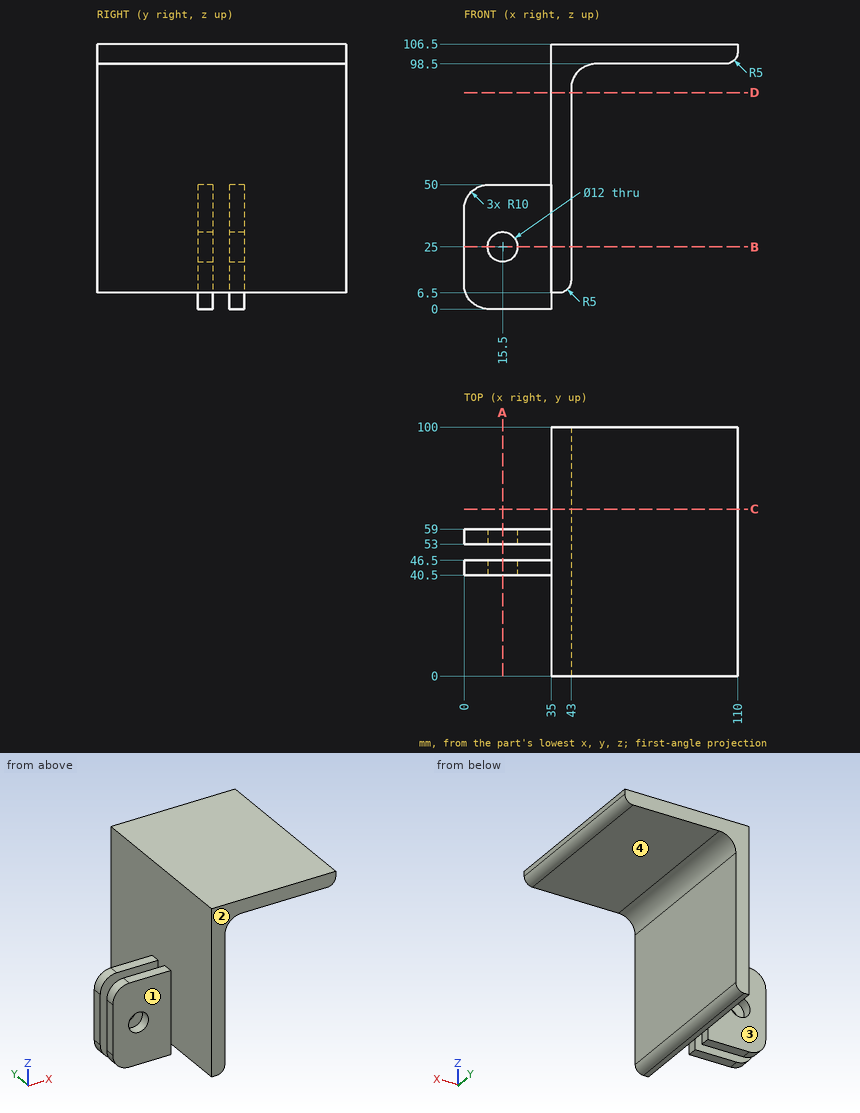
Answer from the drawing. Dimensions are ordinates in mm from the lowest x, y and z of the part. A direction names the side the tool comes from. Give positions to 0.01 mm unless a question says otherwise; leave off trailing zeros. Order: outer loops, then holes, each group sorted by start corner. A loop starts at its lowest first (then second) coordinate and runs counter-clockwise, first axis right, second up. Notation, with made-up numbers: (3.25, -6.75) -> (29.25, -6.75) arc R28 cw to (29.25, 24.25) -> close; hole circle Ø1 at (64.25, 4). An arc over 180 degrees is marked (long way). One line per item, written item: value. Start each with the question number.
(1) Flat-ended cylindrical pins translate along their axes: P1, Ø17.5, axis at x = 20.5, z = 20.5, coming from the -Y side; P2, Ø4, axis at y = 44, z = 34, coming from the +X side; P3, Ø10.5, axis at x = 20.5, z = 31, coming from the +Y side; P4, Ø10, axis at x = 29.5, y = 14, coming from the +Z side. Find the tip coordinate at first contact, or state that the pin passes through.
(2) Straight lines are drawn through the part: L1, parallel to Z at x = 15.5, y = 57; L2, parallel to Y at x = 28.5, z = 23; L3, parallel to Z at x = 96.5, y = 7. For each, find the intervals that lie inside material, in ascending order.
(3) The part is cut by section D-D (z = 87). Determine the outline of the cut face in (x, y), and give its area (3 significant figures).
(4) A tool of negligible diameter and unlimited length cuts with its end or side. For the marked faces 1, 2, 3 and 4, from which of +Z, -Z, +X, -X, +Y, -Y can it reach the whole face along a straight path? Write none if from no direction.
(5) The part is cut by section C-C (y = 67). Determine the outline of the cut face in (x, z), and give its area (3 significant figures).
(6) The part is cut by section B-B (z = 25). Determine the outline of the cut face in (x, y).
(7) The part is cut by section A-A (x = 15.5). Determine the outline of the cut face in (y, z), and give its area (3 significant figures).
Taken from the geometry:
1. P1: y = 40.5
1. P2: x = 43
1. P3: y = 59
1. P4: through
2. L1: 0 to 19, 31 to 50
2. L2: 40.5 to 46.5, 53 to 59
2. L3: 98.5 to 106.5
3. outline: (35, 0) -> (43, 0) -> (43, 100) -> (35, 100) -> close
3. area: 800 mm^2
4. face 1: +Z, -Z, -X, -Y
4. face 2: +Z, -Z, +X, -X, -Y
4. face 3: +Z, -Z, -X, +Y
4. face 4: -Z, +X, +Y, -Y
5. outline: (35, 6.5) -> (38, 6.5) arc R5 ccw to (43, 11.5) -> (43, 88.5) arc R10 cw to (53, 98.5) -> (105, 98.5) arc R5 ccw to (110, 103.5) -> (110, 106.5) -> (35, 106.5) -> close
5. area: 1,350 mm^2
6. outline: (0, 40.5) -> (9.5, 40.5) -> (9.5, 46.5) -> (0, 46.5) -> close; (0, 53) -> (9.5, 53) -> (9.5, 59) -> (0, 59) -> close; (21.5, 40.5) -> (35, 40.5) -> (35, 0) -> (43, 0) -> (43, 100) -> (35, 100) -> (35, 59) -> (21.5, 59) -> (21.5, 53) -> (35, 53) -> (35, 46.5) -> (21.5, 46.5) -> close
7. outline: (40.5, 0) -> (46.5, 0) -> (46.5, 19) -> (40.5, 19) -> close; (40.5, 31) -> (46.5, 31) -> (46.5, 50) -> (40.5, 50) -> close; (53, 0) -> (59, 0) -> (59, 19) -> (53, 19) -> close; (53, 31) -> (59, 31) -> (59, 50) -> (53, 50) -> close
7. area: 456 mm^2
